The listing builds one solid part. Answer for the finished solid, in the listing's coordinates (mm). A direction names the side the tool comes from. Give positions to 0.01 mm unless a question says otherwise; leave off trailing zeros. Order: outer loops, then holes, each group sorted by start corner. A loop starts at its lowest first (then second) coordinate and runs counter-clockwise, first axis right, second up. Notation, with made-up numbers: (28, 24) - (45, 24) arc R13 cw to (45, 28) - close; hole circle Ø10 at (53, 49.25). An arc over 180 degrees is marked (long way). Use a Markdown table: item, result. Add a question column.
1) For faces 4 (the face through (-24.6, -12.1, 81.9)), 5 (the face through (-20.7, -24.6, 72)), 6 (the face through (0, 23.8, 65)), 7 (the face through (-24.61, 11.26, 122.92)), determine the directions among +Z, -Z, +X, -X, +Y, -Y from which every point of the face is accessible in a straight line to the end or side of a thin tool.
2) Straight lines are drawn through the part: line 1 (Y direction, x = -24, z = 7); line 2 (X direction, y = 23, z = 120.5). For each, find the intervals that lie inside material, in ascending order.
3) The mould has two halves that part along Z. Classify faces 1 (the face through (-2, -24, 0)), 2 (the face through (-2, -24, 132)), 3 (the face through (24.61, 12.63, 6.71)): released by +Z, released by -Z, zero draft, split by the parting line, or undercut.
4) Find section D-D, the plane x = -20. Determine the outline of the cut face in (y, z), plus the area to 3 significant figures.
5) Find section A-A, the plane x = 20. Determine the outline of the cut face in (y, z).
6) Find section C-C, the plane z = 39.5. Determine the outline of the cut face in (x, y).
from build123d import *

# Parameters (mm, degrees)
SKETCH1_W                     = 50.8
SKETCH1_H                     = 50.8
SKETCH1_W_2                   = 47.6
SKETCH1_H_2                   = 47.6
BOSS_EXTRUDE1_DEPTH           = 132
M4_CLEARANCE_HOLE1_AT_2_COUNT = 2
M4_CLEARANCE_HOLE1_AT_2_PITCH = 20.8
CIRPATTERN1_COUNT             = 4
CUT_EXTRUDE1_DEPTH            = 5
CUT_EXTRUDE2_DEPTH            = 10


with BuildPart() as part:
    # Sketch1 → Boss-Extrude1 (new body)
    with BuildSketch(Plane.XY):
        Rectangle(SKETCH1_W, SKETCH1_H)
        Rectangle(SKETCH1_W_2, SKETCH1_H_2, mode=Mode.SUBTRACT)
    extrude(amount=BOSS_EXTRUDE1_DEPTH)

    # Sketch5 → M4 Clearance Hole1 (revolve, cut)
    with BuildSketch(Plane(origin=(-25.4, 10.4, 7), x_dir=(0, 0, 1), z_dir=(0, 1, 0))):
        Polygon((0, 0), (0, 12.851936393), (2.25, 11.5), (2.25, 0), align=None)
    m4_clearance_hole1 = revolve(axis=Axis((-31.75, 10.4, 7), (1, 0, 0)), mode=Mode.SUBTRACT)

    # M4 Clearance Hole1 at 2: M4 Clearance Hole1 ×2
    with Locations(*[(0, -i * M4_CLEARANCE_HOLE1_AT_2_PITCH, 0) for i in range(1, M4_CLEARANCE_HOLE1_AT_2_COUNT)]):
        add(m4_clearance_hole1, mode=Mode.SUBTRACT)

    # CirPattern1: M4 Clearance Hole1 ×4 about axis
    cirpattern1_axis = Axis((0, 0, 0), (0, 0, 1))
    for i in range(1, CIRPATTERN1_COUNT):
        add(m4_clearance_hole1.rotate(cirpattern1_axis, i * 360 / CIRPATTERN1_COUNT), mode=Mode.SUBTRACT)

    # CirPattern1 copy 1 sketch → CirPattern1 copy 1 (revolve, cut)
    with BuildSketch(Plane(origin=(10.4, -25.4, 7), x_dir=(0, 0, 1), z_dir=(-1, 0, 0))):
        Polygon((0, 0), (0, 12.851936393), (2.25, 11.5), (2.25, 0), align=None)
    revolve(axis=Axis((10.4, -31.75, 7), (0, 1, 0)), mode=Mode.SUBTRACT)

    # CirPattern1 copy 2 sketch → CirPattern1 copy 2 (revolve, cut)
    with BuildSketch(Plane(origin=(25.4, 10.4, 7), x_dir=(0, 0, 1), z_dir=(0, -1, 0))):
        Polygon((0, 0), (0, 12.851936393), (2.25, 11.5), (2.25, 0), align=None)
    revolve(axis=Axis((31.75, 10.4, 7), (-1, 0, 0)), mode=Mode.SUBTRACT)

    # CirPattern1 copy 3 sketch → CirPattern1 copy 3 (revolve, cut)
    with BuildSketch(Plane(origin=(-10.4, 25.4, 7), x_dir=(0, 0, 1), z_dir=(1, 0, 0))):
        Polygon((0, 0), (0, 12.851936393), (2.25, 11.5), (2.25, 0), align=None)
    revolve(axis=Axis((-10.4, 31.75, 7), (0, -1, 0)), mode=Mode.SUBTRACT)

    # Mirror3: M4 Clearance Hole1 across plane
    add(m4_clearance_hole1.mirror(Plane.XY.offset(66)), mode=Mode.SUBTRACT)

    # Mirror3 copy 1 sketch → Mirror3 copy 1 (revolve, cut)
    with BuildSketch(Plane(origin=(-25.4, -10.4, 125), x_dir=(0, 0, -1), z_dir=(0, 1, 0))):
        Polygon((0, 0), (0, -12.851936393), (2.25, -11.5), (2.25, 0), align=None)
    revolve(axis=Axis((-31.75, -10.4, 125), (-1, 0, 0)), mode=Mode.SUBTRACT)

    # Mirror3 copy 2 sketch → Mirror3 copy 2 (revolve, cut)
    with BuildSketch(Plane(origin=(-10.4, -25.4, 125), x_dir=(0, 0, -1), z_dir=(-1, 0, 0))):
        Polygon((0, 0), (0, -12.851936393), (2.25, -11.5), (2.25, 0), align=None)
    revolve(axis=Axis((-10.4, -31.75, 125), (0, -1, 0)), mode=Mode.SUBTRACT)

    # Mirror3 copy 3 sketch → Mirror3 copy 3 (revolve, cut)
    with BuildSketch(Plane(origin=(25.4, -10.4, 125), x_dir=(0, 0, -1), z_dir=(0, -1, 0))):
        Polygon((0, 0), (0, -12.851936393), (2.25, -11.5), (2.25, 0), align=None)
    revolve(axis=Axis((31.75, -10.4, 125), (1, 0, 0)), mode=Mode.SUBTRACT)

    # Mirror3 copy 4 sketch → Mirror3 copy 4 (revolve, cut)
    with BuildSketch(Plane(origin=(10.4, 25.4, 125), x_dir=(0, 0, -1), z_dir=(1, 0, 0))):
        Polygon((0, 0), (0, -12.851936393), (2.25, -11.5), (2.25, 0), align=None)
    revolve(axis=Axis((10.4, 31.75, 125), (0, 1, 0)), mode=Mode.SUBTRACT)

    # Mirror3 copy 5 sketch → Mirror3 copy 5 (revolve, cut)
    with BuildSketch(Plane(origin=(10.4, -25.4, 125), x_dir=(0, 0, -1), z_dir=(-1, 0, 0))):
        Polygon((0, 0), (0, -12.851936393), (2.25, -11.5), (2.25, 0), align=None)
    revolve(axis=Axis((10.4, -31.75, 125), (0, -1, 0)), mode=Mode.SUBTRACT)

    # Mirror3 copy 6 sketch → Mirror3 copy 6 (revolve, cut)
    with BuildSketch(Plane(origin=(25.4, 10.4, 125), x_dir=(0, 0, -1), z_dir=(0, -1, 0))):
        Polygon((0, 0), (0, -12.851936393), (2.25, -11.5), (2.25, 0), align=None)
    revolve(axis=Axis((31.75, 10.4, 125), (1, 0, 0)), mode=Mode.SUBTRACT)

    # Mirror3 copy 7 sketch → Mirror3 copy 7 (revolve, cut)
    with BuildSketch(Plane(origin=(-10.4, 25.4, 125), x_dir=(0, 0, -1), z_dir=(1, 0, 0))):
        Polygon((0, 0), (0, -12.851936393), (2.25, -11.5), (2.25, 0), align=None)
    revolve(axis=Axis((-10.4, 31.75, 125), (0, 1, 0)), mode=Mode.SUBTRACT)

    # Sketch7 → Cut-Extrude1 (cut)
    with BuildSketch(Plane.ZY.offset(25.4)):
        with BuildLine():
            Line((85, -15.1), (85, -30.1))
            ThreePointArc((85, -30.1), (82, -33.1), (79, -30.1))
            Line((79, -30.1), (79, -15.1))
            ThreePointArc((79, -15.1), (82, -12.1), (85, -15.1))
        make_face()
    extrude(amount=-CUT_EXTRUDE1_DEPTH, mode=Mode.SUBTRACT)

    # Sketch8 → Cut-Extrude2 (cut)
    with BuildSketch(Plane.XZ.offset(25.4)):
        with BuildLine():
            Line((-23.8, 75), (-23.8, 89))
            ThreePointArc((-23.8, 89), (-20.8, 92), (-17.8, 89))
            Line((-17.8, 89), (-17.8, 75))
            ThreePointArc((-17.8, 75), (-20.8, 72), (-23.8, 75))
        make_face()
    extrude(amount=-CUT_EXTRUDE2_DEPTH, mode=Mode.SUBTRACT)


solid = part.part
The answers:
| question | item | result |
|---|---|---|
| 1 | face 4 | -X, -Y |
| 1 | face 5 | -Y |
| 1 | face 6 | +Z, -Z |
| 1 | face 7 | +X, -X |
| 2 | line 1 | -25.4 to -12.65, -8.15 to 8.15, 12.65 to 25.4 |
| 2 | line 2 | -25.4 to -23.8, 23.8 to 25.4 |
| 3 | face 1 | released by -Z |
| 3 | face 2 | released by +Z |
| 3 | face 3 | undercut |
| 4 | outline | (-25.4, 0) - (-23.8, 0) - (-23.8, 72.11) - (-25.4, 72.11) - close; (-25.4, 91.89) - (-23.8, 91.89) - (-23.8, 132) - (-25.4, 132) - close; (23.8, 0) - (25.4, 0) - (25.4, 132) - (23.8, 132) - close |
| 4 | area | 391 mm2 |
| 5 | outline | (-25.4, 0) - (-23.8, 0) - (-23.8, 132) - (-25.4, 132) - close; (23.8, 0) - (25.4, 0) - (25.4, 132) - (23.8, 132) - close |
| 6 | outline | (-25.4, -25.4) - (25.4, -25.4) - (25.4, 25.4) - (-25.4, 25.4) - close; hole (-23.8, -23.8) - (23.8, -23.8) - (23.8, 23.8) - (-23.8, 23.8) - close |
